from build123d import *

# Parameters (mm, degrees)
SKETCH1_W                    = 140
SKETCH1_H                    = 30
SKETCH1_R                    = 4.25
BASE_FLANGE1_DEPTH           = 2
EDGE_FLANGE1_STRIP_W         = 9.4732
EDGE_FLANGE1_STRIP_H         = 2
EDGE_FLANGE1_STRIP_CUT_DEPTH = 30
EDGE_FLANGE1_DEPTH           = 30
SKETCH9_R                    = 4.25
CUT_EXTRUDE1_DEPTH           = 10


# Sheet-metal steps are written as plain solids
with BuildPart() as part:
    # Sketch1 → Base-Flange1 (new body)
    with BuildSketch(Plane.XY):
        with Locations((-9.240282686, 10.521201413)):
            Rectangle(SKETCH1_W, SKETCH1_H)
        with Locations((-65.240282686, 10.521201413)):
            Circle(SKETCH1_R, mode=Mode.SUBTRACT)
    extrude(amount=-BASE_FLANGE1_DEPTH)

    # Edge-Flange1 strip (across the edge) → Edge-Flange1 strip cut (cut)
    with BuildSketch(Plane(origin=(60.759717314, -4.478798587, 0), x_dir=(-1, 0, 0), z_dir=(0, 1, 0))):
        with Locations((-2, -1)):
            Rectangle(EDGE_FLANGE1_STRIP_W, EDGE_FLANGE1_STRIP_H)
    extrude(amount=EDGE_FLANGE1_STRIP_CUT_DEPTH, mode=Mode.SUBTRACT)

    # Edge-Flange1 section (across the edge) → Edge-Flange1 (add)
    with BuildSketch(Plane(origin=(60.759717314, -4.478798587, 0), x_dir=(-1, 0, 0), z_dir=(0, 1, 0))):
        with BuildLine():
            Line((0, 0.7366), (0, 28))
            Line((0, 28), (2, 28))
            Line((2, 28), (2, 0.7366))
            ThreePointArc((2, 0.7366), (2.215745145, 0.215745145), (2.7366, 0))
            Line((2.7366, 0), (2.7366, -2))
            ThreePointArc((2.7366, -2), (0.801531583, -1.198468417), (0, 0.7366))
        make_face()
    extrude(amount=EDGE_FLANGE1_DEPTH)

    # Sketch9 → Cut-Extrude1 (cut)
    with BuildSketch(Plane(origin=(60.759717314, 0, 0), x_dir=(0, 0, -1), z_dir=(1, 0, 0))):
        with Locations((-14, 10.521201413)):
            Circle(SKETCH9_R)
    extrude(amount=-CUT_EXTRUDE1_DEPTH, mode=Mode.SUBTRACT)


solid = part.part
Source: CAD feature listing. Evaluate the final solid. Frame: model axes, mm. A direction names the side the tool comes from. Round coordinates to 2 decimals unless told otherwise and drop trailing zeros. Loops run counter-clockwise (first coordinate to the right, second up) from the corner with the lowest first, then second, coordinate; pieces in that order, holes last.
Q1. Access query for faces 1 (the face through (58.76, 7, 18)), 2 (the face through (59.937, 10.311, -1.22)). Directions: +Z, -Z, +X, -X, +Y, -Y. A direction counts if a zero-diameter tool reaches every point of the face in a straight line with its end or side. Return the directions, or none.
Q2. First-contact query: P1, Ø5, axis at x = -0.5, y = 18, coming from the +Z side; P2, Ø8, axis at y = 4.5, z = 21, coming from the -X side; P3, Ø5, axis at y = 10.52, z = 14, coming from the +X side. Flat tips, straight axial feed; report the tip coordinate or a pass-through.
Q3. Section D-D, the plane z = 8.5. Return loops of the section in (x, y).
Q4. Section A-A, the plane z = 14. Return loops of the section in (x, y).
Q5. Ray query, line 1 (Y direction, x = 59.2, z = 14); line 2 (X direction, y = -0.25, z = 16.5); line 3 (Z direction, x = -71, y = 13.5). Return the intervals inside material, ascending.
Q6. Section B-B, the plane y = 11.75. Return loops of the section in (x, z).
Q7. Section C-C, the plane y = 22.75. Return loops of the section in (x, z), plus the area to 3 significant figures.
Q8. Mould query, pull axis Z, two halves, no side actions, for faces 3 (the face through (-69.486, 10.708, -0.986)), 4 (the face through (-12, 11, 0)), 5 (the face through (59.774, 11.798, 9.946)), 6 (the face through (-12, 11, -2)). Classes: pulls with the +Z half, pulls with the -Z half, needs draft (parallel to the pull), parting line crosses it, or undercut.
Solutions:
1. face 1: +Z, -X, +Y, -Y
1. face 2: -Z, +X, +Y, -Y
2. P1: stops at z = 0
2. P2: stops at x = 58.76
2. P3: passes through
3. outline: (58.76, -4.48) - (60.76, -4.48) - (60.76, 25.52) - (58.76, 25.52) - close
4. outline: (58.76, -4.48) - (60.76, -4.48) - (60.76, 6.27) - (58.76, 6.27) - close; (58.76, 14.77) - (60.76, 14.77) - (60.76, 25.52) - (58.76, 25.52) - close
5. line 1: y = -4.48 to 6.27, 14.77 to 25.52
5. line 2: x = 58.76 to 60.76
5. line 3: z = -2 to 0
6. outline: (-79.24, -2) - (-69.31, -2) - (-69.31, 0) - (-79.24, 0) - close; (-61.17, -2) - (58.02, -2) arc R2.74 ccw to (60.76, 0.74) - (60.76, 9.93) - (58.76, 9.93) - (58.76, 0.74) arc R0.74 cw to (58.02, 0) - (-61.17, 0) - close; (58.76, 18.07) - (60.76, 18.07) - (60.76, 28) - (58.76, 28) - close
7. outline: (-79.24, -2) - (58.02, -2) arc R2.74 ccw to (60.76, 0.74) - (60.76, 28) - (58.76, 28) - (58.76, 0.74) arc R0.74 cw to (58.02, 0) - (-79.24, 0) - close
7. area: 335 mm2
8. face 3: needs draft
8. face 4: pulls with the +Z half
8. face 5: undercut
8. face 6: pulls with the -Z half
